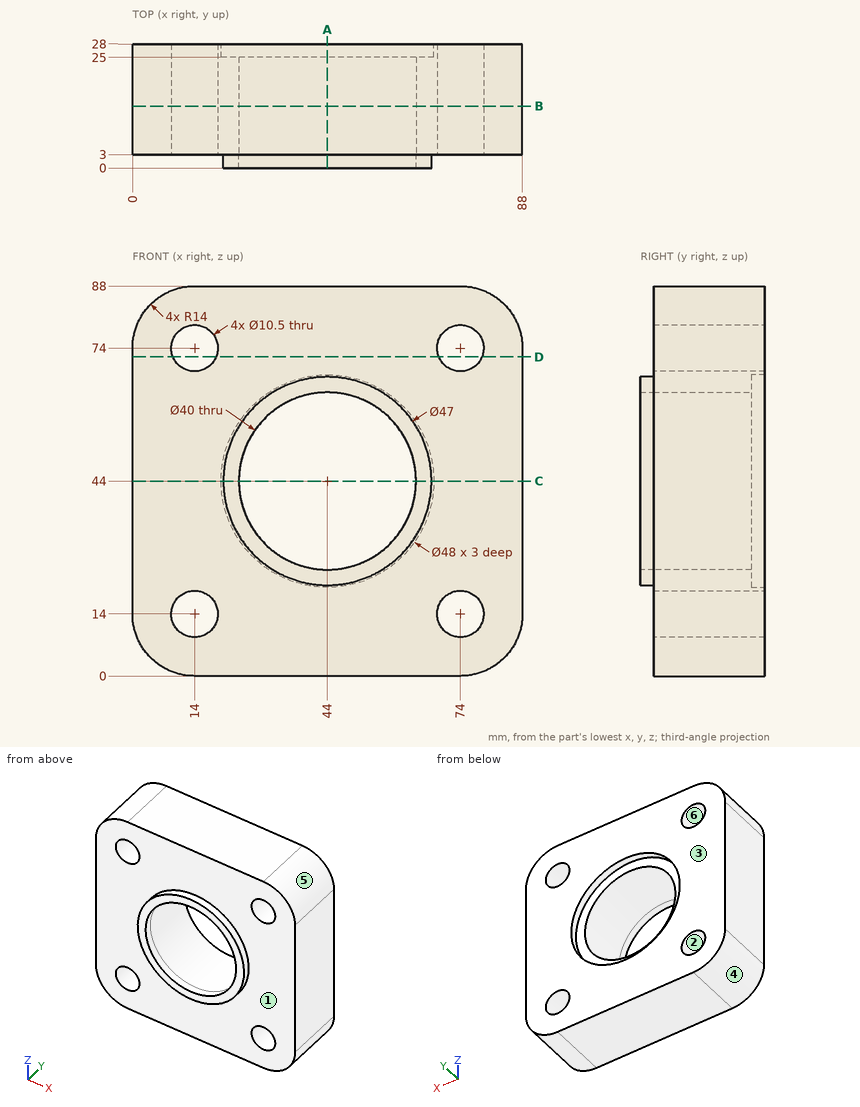
Geometry check sheet. Reference: drawing and pictorial views, mm from the part's lowest x, y, z. A direction names the side the tool comes from. Coordinates: 2 decimals unless noted, no trailing zeros. Loops run counter-clockwise (first coordinate to the right, second up) from the corner with the lowest first, then second, coordinate; pieces in that order, holes last. Notation, with made-up numbers: (74, -28.75) -> (98, -28.75) arc R23 cw to (98, -4.75) -> close; hole circle Ø3 at (19.25, 15.5). An arc over 180 degrees is marked (long way). Write item = value, one per line. Start each with the question number.
1. Tool access check on the marked faces 1 and 2. Record the directions out of +Z, -Z, +X, -X, +Y, -Y that give a thin tool (end or side, any length) a straight path to the whole face; none if there is none.
2. Section check A-A on x = 44. Record the cut outline in (y, z), then the cut area to 3 significant figures.
3. Section check D-D on z = 72. Record the cut outline in (x, y), then the cut area to 3 significant figures.
4. Draft check along X on the marked faces 3, 4, 5 and 6. Enter one of: released by +X, released by -X, zero draft, split by the parting line, or undercut.
5. Section check C-C on z = 44. Record the cut outline in (x, y), then the cut area to 3 significant figures.
6. Section check B-B on y = 14. Record the cut outline in (x, z).
7. Material ranges on line 1 (X direction, y = 19.25, z = 74); line 2 (Z direction, x = 44, y = 19.25); line 3 (X direction, y = 7.75, z = 45), recorded low to high.
8. Depth check by flat-ended pin: P1, Ø3, axis at x = 50, z = 17.5, coming from the -Y side; P2, Ø1.5, axis at y = 19.5, z = 75.5, coming from the +X side; P3, Ø6.5, axis at x = 14, z = 74, coming from the -Y side. Enter the tip coordinate at first touch or a pass-through.
Responses:
q1.face_1 = -Y
q1.face_2 = +Y, -Y
q2.outline = (0, 20.5) -> (3, 20.5) -> (3, 0) -> (28, 0) -> (28, 20) -> (25, 20) -> (25, 24) -> (0, 24) -> close; (0, 64) -> (25, 64) -> (25, 68) -> (28, 68) -> (28, 88) -> (3, 88) -> (3, 67.5) -> (0, 67.5) -> close
q2.area = 1,200 mm2
q3.outline = (0, 3) -> (9.15, 3) -> (9.15, 28) -> (0, 28) -> close; (18.85, 3) -> (69.15, 3) -> (69.15, 28) -> (18.85, 28) -> close; (78.85, 3) -> (88, 3) -> (88, 28) -> (78.85, 28) -> close
q3.area = 1,710 mm2
q4.face_3 = zero draft
q4.face_4 = released by -X
q4.face_5 = released by +X
q4.face_6 = undercut
q5.outline = (0, 3) -> (20.5, 3) -> (20.5, 0) -> (24, 0) -> (24, 25) -> (20, 25) -> (20, 28) -> (0, 28) -> close; (64, 0) -> (67.5, 0) -> (67.5, 3) -> (88, 3) -> (88, 28) -> (68, 28) -> (68, 25) -> (64, 25) -> close
q5.area = 1,200 mm2
q6.outline = (0, 14) arc R14 ccw to (14, 0) -> (74, 0) arc R14 ccw to (88, 14) -> (88, 74) arc R14 ccw to (74, 88) -> (14, 88) arc R14 ccw to (0, 74) -> close; hole circle Ø10.5 at (14, 14); hole circle Ø10.5 at (14, 74); hole circle Ø40 at (44, 44); hole circle Ø10.5 at (74, 14); hole circle Ø10.5 at (74, 74)
q7.line_1 = 0 to 8.75, 19.25 to 68.75, 79.25 to 88
q7.line_2 = 0 to 24, 64 to 88
q7.line_3 = 0 to 24.03, 63.97 to 88
q8.P1 = 3
q8.P2 = 87.98
q8.P3 = through
